The figure shows three views and two pictorial views of one solid part (mm, origin at its lowest corner). Answer the questions. Round coordinates to 2 decimals unless told otherwise and drop trailing zeros. Order: outer loops, then holes, each group sorted by start corner. A loop starts at its lowest first (then second) coordinate and runs counter-clockwise, first axis right, second up. Notation, with made-up numbers: (-4, -22.75) -> (7, -22.75) arc R28 cw to (7, 12.25) -> close; hole circle Ø6 at (-14, -7). An arc over 180 degrees is marked (long way). Return JSON: item names as keys, results as strings. Group by question number.
(1) The part is cut by section C-C (x = 10.25). Determine the outline of the cut face in (y, z) (1 decimal).
(2) Consider line 1 (X direction, y = 1, z = 0.7) (1 decimal); line 2 (Y direction, x = 13.25, z = 0.6) (1 decimal); line 3 (Y direction, x = 5, z = 0.5) (1 decimal). Determine where each line is inside the solid, lowest interval first. Write a range as [from, to].
(3) The part is cut by section A-A (y = 9.25). Determine the outline of the cut face in (x, z) (1 decimal).
(4) The part is cut by section B-B (z = 0.2). Count the separate pieces of the cut face and the enclosed holes in it.
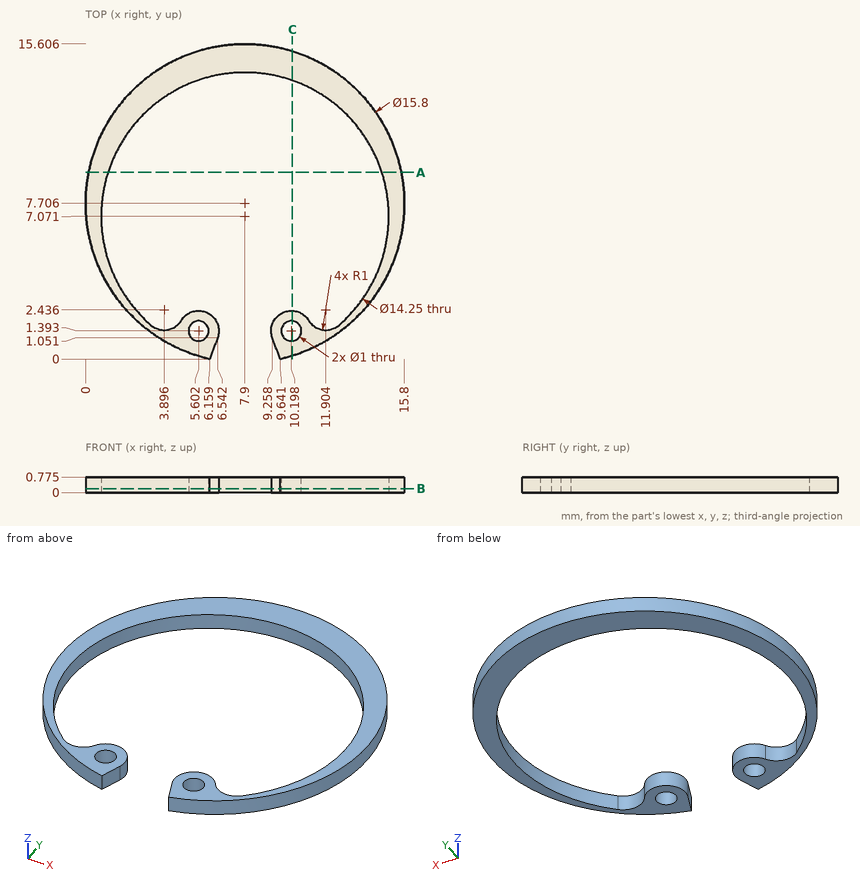
Answer below:
{
 "1": {"outline": "(0.2, 0) -> (0.9, 0) -> (0.9, 0.8) -> (0.2, 0.8) -> close; (1.9, 0) -> (2.4, 0) -> (2.4, 0.8) -> (1.9, 0.8) -> close; (13.8, 0) -> (15.2, 0) -> (15.2, 0.8) -> (13.8, 0.8) -> close"},
 "2": {"line 1": "x = [3.7, 5.3], [5.9, 6.5], [9.3, 9.9], [10.5, 12.1]", "line 2": "y = [1.9, 2.4], [11.8, 13.5]", "line 3": "y = [0.4, 2.2], [13.6, 15.1]"},
 "3": {"outline": "(0.2, 0) -> (1.1, 0) -> (1.1, 0.8) -> (0.2, 0.8) -> close; (14.7, 0) -> (15.6, 0) -> (15.6, 0.8) -> (14.7, 0.8) -> close"},
 "4": {"separate pieces": "1", "enclosed holes": "2"}
}
